Build history of the part. All positions in model axes, mm. Round coordinates to 2 decimals unless told otherwise and drop trailing zeros. Write each loop counter-clockwise with the first axis right and the second up, starting at its lowest first coordinate (ties: lowest second). Pieces come first, ordered by that corner, then holes. Notation, with made-up numbers: (42, 40) - (95, 40) arc R21 cw to (95, 62) - close; hole circle Ø11 at (-6.75, -35). An arc over 180 degrees is marked (long way). Write each question's results on one line, items separated by ' | '.
from build123d import *

# Parameters (mm, degrees)
F1_DEPTH = 5.08


with BuildPart() as f1:
    # F0 (on Right) → F1 (new body)
    with BuildSketch(Plane.YZ):
        Polygon((-25.4, 0.091885), (0, 0.091885), (25.4, 0.091885), (25.4, -4.988115), (63.5, -4.988115), (63.5, 0.091885), (88.9, 0), (88.9, 6.436423), (88.9, 108.036423), (-88.9, 108.036423), (-88.9, 6.436423), (-88.9, 0), (-63.5, 0.091885), (-63.5, -4.988115), (-25.4, -4.988115), align=None)
    extrude(amount=F1_DEPTH)


solid = f1.part
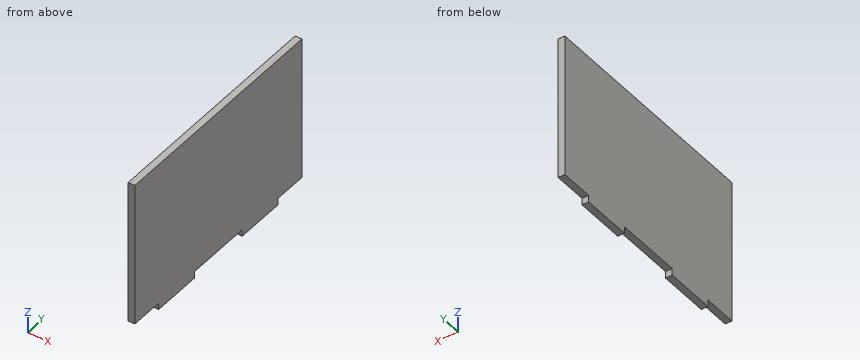
(1) Slice it at A-A, the plane x = 3.35. Write the cut outline in (y, z), and give its area (3 significant figures).
Worked answers:
outline: (-88.9, 0) - (-63.5, 0.09) - (-63.5, -4.99) - (-25.4, -4.99) - (-25.4, 0.09) - (25.4, 0.09) - (25.4, -4.99) - (63.5, -4.99) - (63.5, 0.09) - (88.9, 0) - (88.9, 108.04) - (-88.9, 108.04) - close | area: 19,600 mm2
(2) Drill centre lines: probe 1 along Z at (x, y) = (3.35, 17); probe 2 along Z at (x, y) = (2.1, -77). Where is each one in solid material? Low to high. Write a range as [from, to].
Worked answers:
probe 1: z = [0.09, 108.04] | probe 2: z = [0.04, 108.04]
(3) Slice it at B-B, the plane y = 0. Write the cut outline in (x, z), and give its area (3 significant figures).
Worked answers:
outline: (0, 0.09) - (5.08, 0.09) - (5.08, 108.04) - (0, 108.04) - close | area: 548 mm2
(4) Slice it at C-C, the plane y = 75. Write the cut outline in (x, z).
Worked answers:
outline: (0, 0.05) - (5.08, 0.05) - (5.08, 108.04) - (0, 108.04) - close
(5) Flat gauge pins, fed straight in: pin 1 Ø2.5 at (x, y) = (1.5, 2) entering from -Z; pin 2 Ø1.5 at (x, z) = (1.5, -1.5) entering from +Y; pin 3 Ø2.5 at (x, z) = (2.5, -2) entering from -Y. Where does each tip first touch, or does it go through?
Worked answers:
pin 1: stops at z = 0.09 | pin 2: stops at y = 63.5 | pin 3: stops at y = -63.5
